```python
from build123d import *

# Parameters (mm, degrees)
SKETCH1_W           = 61
SKETCH1_H           = 12
SKETCH1_R           = 3.25
BOSS_EXTRUDE1_DEPTH = 4
BOSS_EXTRUDE2_START = -20
BOSS_EXTRUDE2_DEPTH = 21
CUT_EXTRUDE1_REACH  = 82.162


with BuildPart() as part:
    # Sketch1 → Boss-Extrude1 (new body)
    with BuildSketch(Plane.XY):
        with Locations((30.5, 6)):
            Rectangle(SKETCH1_W, SKETCH1_H)
        with Locations((7.5, 6)):
            Circle(SKETCH1_R, mode=Mode.SUBTRACT)
        with Locations((53.5, 6)):
            Circle(SKETCH1_R, mode=Mode.SUBTRACT)
    extrude(amount=BOSS_EXTRUDE1_DEPTH)

    # Sketch3 → Boss-Extrude2 (add)
    with BuildSketch(Plane.ZY.offset(BOSS_EXTRUDE2_START)):
        Polygon((4, 12), (4, 28), (41, 28), (41, 32), (0, 32), (0, 12), align=None)
    extrude(amount=-BOSS_EXTRUDE2_DEPTH)

    # Sketch4 → Cut-Extrude1 (cut, up to next)
    with BuildSketch(Plane(origin=(0, 32, 0), x_dir=(1, 0, 0), z_dir=(0, 1, 0)), mode=Mode.PRIVATE) as cut_extrude1_sk1:
        with BuildLine():
            Line((36, -22.35), (36, -37.35))
            ThreePointArc((36, -37.35), (35.35, -38), (34.7, -37.35))
            Line((34.7, -37.35), (34.7, -22.35))
            ThreePointArc((34.7, -22.35), (35.35, -21.7), (36, -22.35))
        make_face()
    cut_extrude1_tool1 = extrude(cut_extrude1_sk1.sketch, amount=-CUT_EXTRUDE1_REACH, mode=Mode.PRIVATE) & part.part
    # Sketch4 → Cut-Extrude1 (cut, up to next)
    with BuildSketch(Plane(origin=(0, 32, 0), x_dir=(1, 0, 0), z_dir=(0, 1, 0)), mode=Mode.PRIVATE) as cut_extrude1_sk2:
        with BuildLine():
            Line((26.3, -22.35), (26.3, -37.35))
            ThreePointArc((26.3, -37.35), (25.65, -38), (25, -37.35))
            Line((25, -37.35), (25, -22.35))
            ThreePointArc((25, -22.35), (25.65, -21.7), (26.3, -22.35))
        make_face()
    cut_extrude1_tool2 = extrude(cut_extrude1_sk2.sketch, amount=-CUT_EXTRUDE1_REACH, mode=Mode.PRIVATE) & part.part
    add(cut_extrude1_tool1.solids().sort_by_distance((35.35, 32, 29.85))[0], mode=Mode.SUBTRACT)
    add(cut_extrude1_tool2.solids().sort_by_distance((25.65, 32, 29.85))[0], mode=Mode.SUBTRACT)


solid = part.part
```
Input: part model. Units: mm. Frame: model coordinates. A direction names the side the tool comes from. Coordinates: 2 decimals unless noted, no trailing zeros. Write each loop counter-clockwise with the first axis right and the second up, starting at its lowest first coordinate (ties: lowest second). Pieces come first, ordered by that corner, then holes. Notation, with made-up numbers: M 46.5,-7.75 L 57.5,-7.75 A26 ccw 57.5,11.25 Z; hole C -20,24 d2. An arc over 180 degrees is marked long. Use one line per item in the form item = value.
Q1. Section C-C (z = 34.5). Return loops of the section in (x, y).
Answer below:
outline = M 20,28 L 25,28 L 25,32 L 20,32 Z; M 26.3,28 L 34.7,28 L 34.7,32 L 26.3,32 Z; M 36,28 L 41,28 L 41,32 L 36,32 Z
Q2. Material intervals for probe 1 along Y at (x, z) = (53.5, 1.3); probe 2 along Z at (x, y) = (24, 3.5); probe 3 along Y at (x, z) = (40.5, 38.5), sorted ascending. Write a range as from..to.
Answer below:
probe_1 = 0..2.75, 9.25..12
probe_2 = 0..4
probe_3 = 28..32
Q3. Section A-A (x = 35.35). Return loops of the section in (y, z), plus the area to 3 significant figures.
Answer below:
outline = M 0,0 L 32,0 L 32,21.7 L 28,21.7 L 28,4 L 0,4 Z; M 28,38 L 32,38 L 32,41 L 28,41 Z
area = 211 mm²
Q4. Draft query along X for faces 1 (the face through (35.4, 30, 38)), 2 (the face through (20, 29, 16)), 3 (the face through (61, 6, 2)), 4 (the face through (30, 30, 41)). Return one class per face: released by +X, released by -X, zero draft, split by the parting line, or undercut.
Answer below:
face_1 = undercut
face_2 = released by -X
face_3 = released by +X
face_4 = zero draft
Q5. Section B-B (y = 6). Return loops of the section in (x, z).
Answer below:
outline = M 0,0 L 4.25,0 L 4.25,4 L 0,4 Z; M 10.75,0 L 50.25,0 L 50.25,4 L 10.75,4 Z; M 56.75,0 L 61,0 L 61,4 L 56.75,4 Z
Q6. First-contact query: pin 1 (4.5 mm diameter, centred on y = 30.5, z = 27.5, fed in from -X); pin 2 (4.5 mm diameter, centred on x = 53, z = 2.5, fed in from +Y); pin 3 (3 mm diameter, centred on y = 29, z = 32.5, fed in from +X). Flat tips, straight axial feed; report the tip coordinate or a pass-through.
Answer below:
pin_1 = 20
pin_2 = 12
pin_3 = 41
Q7. Section D-D (x = 7.5). Return loops of the section in (y, z).
Answer below:
outline = M 0,0 L 2.75,0 L 2.75,4 L 0,4 Z; M 9.25,0 L 12,0 L 12,4 L 9.25,4 Z
Q8. Set-up query: faces 5 (the face through (41, 29, 16)), 6 (the face through (30, 28, 22)), 7 (the face through (26.3, 30, 30)). Return all of +Z, -Z, +X, -X, +Y, -Y with unobstructed straight access to the full face (end or side cutting, diameter ignored); none if empty.
Answer below:
face_5 = +Z, -Z, +X, +Y
face_6 = +Z, +X, -X, -Y
face_7 = +Y, -Y
